Autodesk Fusion 360 part; units mm, degrees
sketch "Sketch1" plane through (0, 0, 0) normal (0, 1, 0) x (1, 0, 0)
  line L0 (0, 0) -> (76.2, 0)
  line L1 (76.2, 0) -> (76.2, 266.7)
  line L2 (76.2, 266.7) -> (0, 266.7)
  line L3 (0, 266.7) -> (0, 0)
extrude "Extrude1" add sketch "Sketch1" along normal blind 6.35
sketch "Sketch2" plane through (0, 6.35, 0) normal (0, 1, 0) x (-1, 0, 0)
  line L0 (0, -266.7) -> (0, 0)
  line L1 (0, 0) -> (-76.2, 0)
  line L2 (-76.2, 0) -> (-76.2, -266.7)
  line L3 (-76.2, -266.7) -> (0, -266.7)
  circle A0 centre (-25.4, -12.7) radius 1.27
  dimension "d3" = 2.54
extrude "Extrude2" cut sketch "Sketch2" against normal blind 6.35 contours A0
sketch "Sketch3" plane through (0, 6.35, 0) normal (0, 1, 0) x (-1, 0, 0)
  circle A0 centre (-25.4, -12.7) radius 1.27
  line L0 (0, -266.7) -> (0, 0)
  line L1 (0, 0) -> (-76.2, 0)
  line L2 (-76.2, 0) -> (-76.2, -266.7)
  line L3 (-76.2, -266.7) -> (0, -266.7)
  circle A1 centre (-50.8, -12.7) radius 1.27
  circle A2 centre (-25.4, -254) radius 1.27
  circle A3 centre (-50.8, -254) radius 1.27
  dimension "d6" = 2.54
  dimension "d7" = 2.54
  dimension "d8" = 2.54
extrude "Extrude3" cut sketch "Sketch3" against normal blind 6.35 contours A1 | A2 | A3
sketch "Sketch4" plane through (0, 6.35, 0) normal (0, 1, 0) x (-1, 0, 0)
  circle A0 centre (-50.8, -12.7) radius 1.27
  circle A1 centre (-50.8, -254) radius 1.27
  circle A2 centre (-25.4, -254) radius 1.27
  circle A3 centre (-25.4, -12.7) radius 1.27
  line L0 (0, -266.7) -> (0, 0)
  line L1 (0, 0) -> (-76.2, 0)
  line L2 (-76.2, 0) -> (-76.2, -266.7)
  line L3 (-76.2, -266.7) -> (0, -266.7)
  line L4 (-25.4, -146.05) -> (-50.8, -146.05)
  line L5 (-50.8, -146.05) -> (-50.8, -120.65)
  line L6 (-50.8, -120.65) -> (-25.4, -120.65)
  line L7 (-25.4, -120.65) -> (-25.4, -146.05)
  dimension "d11" = 25.4
  dimension "d12" = 25.4
extrude "Extrude4" cut sketch "Sketch4" against normal blind 6.35 contours L4 L5 L6 L7
sketch "Sketch5" plane through (0, 6.35, 0) normal (0, 1, 0) x (-1, 0, 0)
  line L0 (-50.8, -146.05) -> (-50.8, -120.65)
  line L1 (-50.8, -120.65) -> (-25.4, -120.65)
  line L2 (-25.4, -120.65) -> (-25.4, -146.05)
  line L3 (-25.4, -146.05) -> (-50.8, -146.05)
  circle A0 centre (-50.8, -12.7) radius 1.27
  circle A1 centre (-50.8, -254) radius 1.27
  circle A2 centre (-25.4, -254) radius 1.27
  circle A3 centre (-25.4, -12.7) radius 1.27
  line L4 (0, -266.7) -> (0, 0)
  line L5 (0, 0) -> (-76.2, 0)
  line L6 (-76.2, 0) -> (-76.2, -266.7)
  line L7 (-76.2, -266.7) -> (0, -266.7)
  line L8 (-50.8, -146.05) -> (-53.34, -146.05)
  line L9 (-53.34, -146.05) -> (-53.34, -120.65)
  line L10 (-53.34, -120.65) -> (-50.8, -120.65)
  line L11 (-50.8, -120.65) -> (-50.8, -146.05)
  line L12 (-22.86, -148.59) -> (-53.34, -148.59)
  line L13 (-53.34, -148.59) -> (-53.34, -146.05)
  line L14 (-53.34, -146.05) -> (-22.86, -146.05)
  line L15 (-22.86, -146.05) -> (-22.86, -148.59)
  line L16 (-22.86, -146.05) -> (-25.4, -146.05)
  line L17 (-25.4, -146.05) -> (-25.4, -118.11)
  line L18 (-25.4, -118.11) -> (-22.86, -118.11)
  line L19 (-22.86, -118.11) -> (-22.86, -146.05)
  line L20 (-25.4, -118.11) -> (-53.34, -118.11)
  line L21 (-53.34, -118.11) -> (-53.34, -120.65)
  line L22 (-53.34, -120.65) -> (-25.4, -120.65)
  line L23 (-25.4, -120.65) -> (-25.4, -118.11)
extrude "Extrude5" cut sketch "Sketch5" against normal blind 6.35 contours L0 L8 L9 L10 L11 L14 L22 | L3 L8 L12 L13 L14 L15 L16 | L1 L10 L17 L20 L21 L22 L23 | L2 L14 L16 L17 L18 L19 L23
For this review, take the finished solid that the model builds, in its own axes (mm). A direction names the side the tool comes from. Round coordinates to 2 decimals unless told otherwise and drop trailing zeros. Order: outer loops, then holes, each group sorted by start corner. A loop starts at its lowest first (then second) coordinate and runs counter-clockwise, first axis right, second up. Notation, with made-up numbers: (-30, 0) -> (-16, 0) arc R17 cw to (-16, 6) -> close; hole circle Ø6 at (23, -7). An arc over 180 degrees is marked (long way). Put each result on its own line as item: value.
Q1. Machinability: for faces 1 (the flat face through (22.86, 3, -133)), 2 (the flat face through (54, 6.35, -135)), which of the approach directions +Z, -Z, +X, -X, +Y, -Y give a long, thin tool a straight path to every point of the face, cutting with its end or side? Answer none if there is none.
Check result:
face 1: +Y, -Y
face 2: +Z, -Z, +X, -X, +Y
Q2. Add section B-B on x = 44.5. Write out the cut boundary in (y, z).
Check result:
outline: (0, -266.7) -> (6.35, -266.7) -> (6.35, -148.59) -> (0, -148.59) -> close; (0, -118.11) -> (6.35, -118.11) -> (6.35, 0) -> (0, 0) -> close
Q3. Mouldability with a two-part tool opening along Z and no side actions: class faces 3 (the flat face through (38, 3, -148.59)), 4 (the flat face through (38, 3, -118.11)), 5 (the flat face through (0, 3, -135)), 6 (the flat face through (38, 3, 0)) as pulls with the +Z half, pulls with the -Z half, needs draft (parallel to the pull), parting line crosses it, or undercut.
Check result:
face 3: undercut
face 4: undercut
face 5: needs draft
face 6: pulls with the +Z half
Q4. Insertion check: pin 1 Ø2 at (x, z) = (50.8, -12.7) entering from -Y. The pin has a flat end and moves straight along its axis. Give the tip position at first contact, or say it passes through.
Check result:
pin 1: through
Q5. For probe 1 along Z at (x, y) = (50.8, 5); probe 2 along Z at (x, y) = (24.5, 1.5); probe 3 along Z at (x, y) = (36, 5.75), list the stretches that pass through material, from the lowest coordinate up. Write a range as [from, to].
Check result:
probe 1: [-266.7, -255.27], [-252.73, -148.59], [-118.11, -13.97], [-11.43, 0]
probe 2: [-266.7, -254.9], [-253.1, -148.59], [-118.11, -13.6], [-11.8, 0]
probe 3: [-266.7, -148.59], [-118.11, 0]
Q6. Add section A-A on y = 2. Write out the cut boundary in (x, z).
Check result:
outline: (0, -266.7) -> (76.2, -266.7) -> (76.2, 0) -> (0, 0) -> close; hole (22.86, -148.59) -> (53.34, -148.59) -> (53.34, -118.11) -> (22.86, -118.11) -> close; hole circle Ø2.54 at (25.4, -254); hole circle Ø2.54 at (25.4, -12.7); hole circle Ø2.54 at (50.8, -254); hole circle Ø2.54 at (50.8, -12.7)
